from build123d import *

# Parameters (mm, degrees)
SKETCH1_R           = 10
BOSS_EXTRUDE1_DEPTH = 10
SKETCH1_3_R         = 1.15
BOSS_EXTRUDE2_DEPTH = 2
CUT_EXTRUDE1_START  = -10
SKETCH1_4_R         = 1.5
CUT_EXTRUDE1_DEPTH  = 5


with BuildPart() as part:
    # Sketch1 → Boss-Extrude1 (new body)
    with BuildSketch(Plane(origin=(0, 0, 0), x_dir=(1, 0, 0), z_dir=(0, 1, 0))):
        Circle(SKETCH1_R)
    extrude(amount=-BOSS_EXTRUDE1_DEPTH)

    # Sketch1<3> → Boss-Extrude2 (add)
    with BuildSketch(Plane(origin=(0, 0, 0), x_dir=(1, 0, 0), z_dir=(0, 1, 0))):
        Circle(SKETCH1_3_R)
    extrude(amount=BOSS_EXTRUDE2_DEPTH)

    # Sketch1<4> → Cut-Extrude1 (cut)
    with BuildSketch(Plane(origin=(0, 0, 0), x_dir=(1, 0, 0), z_dir=(0, 1, 0)).offset(CUT_EXTRUDE1_START)):
        with Locations((6.495190528, -3.75)):
            Circle(SKETCH1_4_R)
        with Locations((-6.495190528, -3.75)):
            Circle(SKETCH1_4_R)
        with Locations((0, 7.5)):
            Circle(SKETCH1_4_R)
    extrude(amount=CUT_EXTRUDE1_DEPTH, mode=Mode.SUBTRACT)


solid = part.part
The model under review builds one solid part; all positions refer to its coordinate system, in mm. A direction names the side the tool comes from. Coordinates: 2 decimals unless noted, no trailing zeros. Loops run counter-clockwise (first coordinate to the right, second up) from the corner with the lowest first, then second, coordinate; pieces in that order, holes last. Notation, with made-up numbers: (37.5, 2) -> (93.5, 2) arc R20 ccw to (93.5, 11) -> close; hole circle Ø9 at (-16, -21). An arc over 180 degrees is marked (long way). Use a Markdown table: item, result. Add a question column.
1. Add section C-C on y = -7.25. Write out the cut boundary in (x, z), plus the area to 3 significant figures.
2. Add section B-B on z = 0. Write out the cut boundary in (x, y).
3. Machinability: for faces 1 (the face through (-0.91, 0.99, 0.7)), 2 (the face through (6, -5, 4)), 3 (the face through (0, -10, 0)), which of the approach directions +Z, -Z, +X, -X, +Y, -Y give a long, thin tool a straight path to every point of the face, cutting with its end or side? Answer none if there is none.
4. Add section D-D on y = -3.75. Write out the cut boundary in (x, z), plus the area to 3 significant figures.
5. Clearance check with flat-ended pins moving along their axes: pin 1 Ø1.8 at (x, z) = (-6.5, 3.75) entering from -Y; pin 2 Ø3.5 at (x, z) = (6.5, 3.5) entering from -Y; pin 3 Ø1 at (x, y) = (-4.5, -6.5) entering from +Z; pin 4 Ø1 at (x, y) = (2.5, -1.5) entering from +Z. State where each tip first meets the part, or that it passes through.
6. Add section A-A on x = 0. Write out the cut boundary in (y, z), plus the area to 3 significant figures.
7. To check wall thickness, follow line 1 (Y direction, x = 4, z = -5.5); line 2 (Z direction, x = 0, y = -6.95); line 3 (X direction, y = -8, z = 3.75). State the ranges of each line that lie inside material, in increasing order.
8. Draft analysis for pull direction Z (two halves, no side actions). For faces 4 (the face through (0, -8, -6)), 5 (the face through (-7, -5, 4)), 6 (the face through (0, 2, 0)), 7 (the face through (-2.17, -4.93, 9.76)), state which applies: pulls with the +Z half, pulls with the -Z half, needs draft (parallel to the pull), parting line crosses it, or undercut.
Returned:
| question | item | result |
|---|---|---|
| 1 | outline | circle Ø20 at (0, 0); hole circle Ø3 at (-6.5, 3.75); hole circle Ø3 at (0, -7.5); hole circle Ø3 at (6.5, 3.75) |
| 1 | area | 293 mm² |
| 2 | outline | (-10, -10) -> (10, -10) -> (10, 0) -> (1.15, 0) -> (1.15, 2) -> (-1.15, 2) -> (-1.15, 0) -> (-10, 0) -> close |
| 3 | face 1 | +Y |
| 3 | face 2 | -Y |
| 3 | face 3 | +Z, -Z, +X, -X, -Y |
| 4 | outline | circle Ø20 at (0, 0) |
| 4 | area | 314 mm² |
| 5 | pin 1 | stops at y = -5 |
| 5 | pin 2 | stops at y = -10 |
| 5 | pin 3 | stops at z = 9.17 |
| 5 | pin 4 | stops at z = 9.8 |
| 6 | outline | (-10, -10) -> (0, -10) -> (0, -1.15) -> (2, -1.15) -> (2, 1.15) -> (0, 1.15) -> (0, 10) -> (-10, 10) -> (-10, -6) -> (-5, -6) -> (-5, -9) -> (-10, -9) -> close |
| 6 | area | 190 mm² |
| 7 | line 1 | y = -10 to 0 |
| 7 | line 2 | z = -10 to -9, -6 to 10 |
| 7 | line 3 | x = -9.27 to -8, -5 to 5, 8 to 9.27 |
| 8 | face 4 | undercut |
| 8 | face 5 | undercut |
| 8 | face 6 | needs draft |
| 8 | face 7 | parting line crosses it |
